Build history of the part. All positions in model axes, mm. A direction names the side the tool comes from. Round coordinates to 2 decimals unless told otherwise and drop trailing zeros. Write each loop counter-clockwise with the first axis right and the second up, starting at its lowest first coordinate (ties: lowest second). Pieces come first, ordered by that corner, then holes.
from build123d import *

# Parameters (mm, degrees)
F0_R     = 8.255
F1_DEPTH = 12.7
F3_DEPTH = 3.175
F4_R     = 6.223
F5_DEPTH = 19.05
F6_SIZE  = 1.5875


with BuildPart() as f1:
    # F0 (on Top) → F1 (new body)
    with BuildSketch(Plane.XY):
        with BuildLine():
            Line((19.05, 10.16), (0, 10.16))
            ThreePointArc((0, 10.16), (-10.16, 0), (0, -10.16))
            Line((0, -10.16), (19.05, -10.16))
            ThreePointArc((19.05, -10.16), (29.21, 0), (19.05, 10.16))
        make_face()
        Circle(F0_R, mode=Mode.SUBTRACT)
        with Locations((19.05, 0)):
            Circle(F0_R, mode=Mode.SUBTRACT)
    extrude(amount=F1_DEPTH)

    # F2 (on face) → F3 (join)
    with BuildSketch(Plane.XY.offset(12.7)):
        with BuildLine():
            Line((19.05, 10.16), (0, 10.16))
            ThreePointArc((0, 10.16), (-10.16, 0), (0, -10.16))
            Line((0, -10.16), (19.05, -10.16))
            ThreePointArc((19.05, -10.16), (29.21, 0), (19.05, 10.16))
        make_face()
    extrude(amount=F3_DEPTH)

    # F4 (on face) → F5 (join)
    with BuildSketch(Plane.XY.offset(15.875)):
        with Locations((9.525, 0)):
            Circle(F4_R)
    extrude(amount=F5_DEPTH)

    # F6
    f6_edges = [f1.edges().sort_by_distance(p)[0] for p in [
        (3.302, 0, 34.925),
    ]]
    chamfer(f6_edges, length=F6_SIZE)


solid = f1.part
1) Slice it at C-C (x = -7). Write the cut outline in (y, z) (1 decimal).
Results:
outline: (-7.4, 0) - (-4.4, 0) - (-4.4, 12.7) - (4.4, 12.7) - (4.4, 0) - (7.4, 0) - (7.4, 15.9) - (-7.4, 15.9) - close
2) Slice it at B-B (z = 28.5). Write the cut outline in (x, y) (3 decimals).
Results:
outline: circle Ø12.446 at (9.525, 0)
3) Wall check: L1, parallel to Y at x = 19.05, z = 8.75 (3 decimals); L2, parallel to X at y = 1.75, z = 11; L3, parallel to Z at x = -3, y = -0.5 (3 decimals). Give the ranges that are in metal, low to high.
Results:
L1: y = -10.16 to -8.255, 8.255 to 10.16
L2: x = -10.01 to -8.07, 8.07 to 10.98, 27.12 to 29.06
L3: z = 12.7 to 15.875
4) Mould opens along Y. For faces 4 (the flat face through (19, 0, 12.7)), 5 (the flat face through (9, -10.16, 8)), 6 (the flat face through (9, 0, 34.925)) say: released by +Y, released by -Y, zero draft, split by the parting line, or undercut.
Results:
face 4: undercut
face 5: released by -Y
face 6: zero draft
5) Slice it at D-D (y = 7.25). Write the cut outline in (x, z) (3 decimals), plus the area to 3 significant figures.
Results:
outline: (-7.118, 0) - (-3.947, 0) - (-3.947, 12.7) - (3.947, 12.7) - (3.947, 0) - (15.103, 0) - (15.103, 12.7) - (22.997, 12.7) - (22.997, 0) - (26.168, 0) - (26.168, 15.875) - (-7.118, 15.875) - close
area: 328 mm2
6) Pin check, flat tips, straight feed: pin 1 Ø5 at (x, y) = (21, -3) entering from -Z; pin 2 Ø1 at (y, z) = (4.5, 11) entering from +X; pin 3 Ø8 at (x, y) = (-5, 1.5) entering from +Z (3 decimals). Stop position of each tip, or through.
Results:
pin 1: stops at z = 12.7
pin 2: stops at x = 28.39
pin 3: stops at z = 15.875
7) Which spindle directions (+Z, -Z, +X, -X, +Y, -Y) get a long thin tool onto all of the face, cutting with end or side? Do faces 1 (the cylindrical face through (-10.158, 0.223, 7.826)), 2 (the cylindrical face through (7.874, 2.48, 6.261)), 3 (the cylindrical face through (15.46, 1.87, 24.48)). Say none if no direction does.
Results:
face 1: +Z, -Z, -X
face 2: -Z
face 3: +Z
8) Slice it at A-A (y = 0). Write the cut outline in (x, z) (1 decimal).
Results:
outline: (-10.2, 0) - (-8.3, 0) - (-8.3, 12.7) - (8.3, 12.7) - (8.3, 0) - (10.8, 0) - (10.8, 12.7) - (27.3, 12.7) - (27.3, 0) - (29.2, 0) - (29.2, 15.9) - (15.7, 15.9) - (15.7, 33.3) - (14.2, 34.9) - (4.9, 34.9) - (3.3, 33.3) - (3.3, 15.9) - (-10.2, 15.9) - close
